Geometry: see drawing. Coordinates: mm, zero at the bounding-box minimum. Round coordinates to 2 decimals unless told otherwise and drop trailing zeros. Loops run counter-clockwise (first coordinate to the right, second up) from the corner with the lowest first, then second, coordinate; pieces in that order, holes last. Notation, with made-up numbers: (89, 82.5) - (139, 82.5) arc R29 ccw to (139, 113.5) - close; hole circle Ø11 at (18, 25). An arc over 180 degrees is marked (long way). Write item = value, one per line. Start each with the question number.
Item 1: Section B-B (x = 14.5). Return loops of the section in (y, z).
Item 2: Section A-A (y = 11). Return loops of the section in (x, z), plus the area to 3 significant figures.
Item 3: Line query: line 1 (Z direction, x = 19, y = 38); line 2 (Z direction, x = 9, y = 12) (1 decimal); line 3 (X direction, y = 4, z = 353). Output: solid intervals per line, ascending. Write a range as from..to.
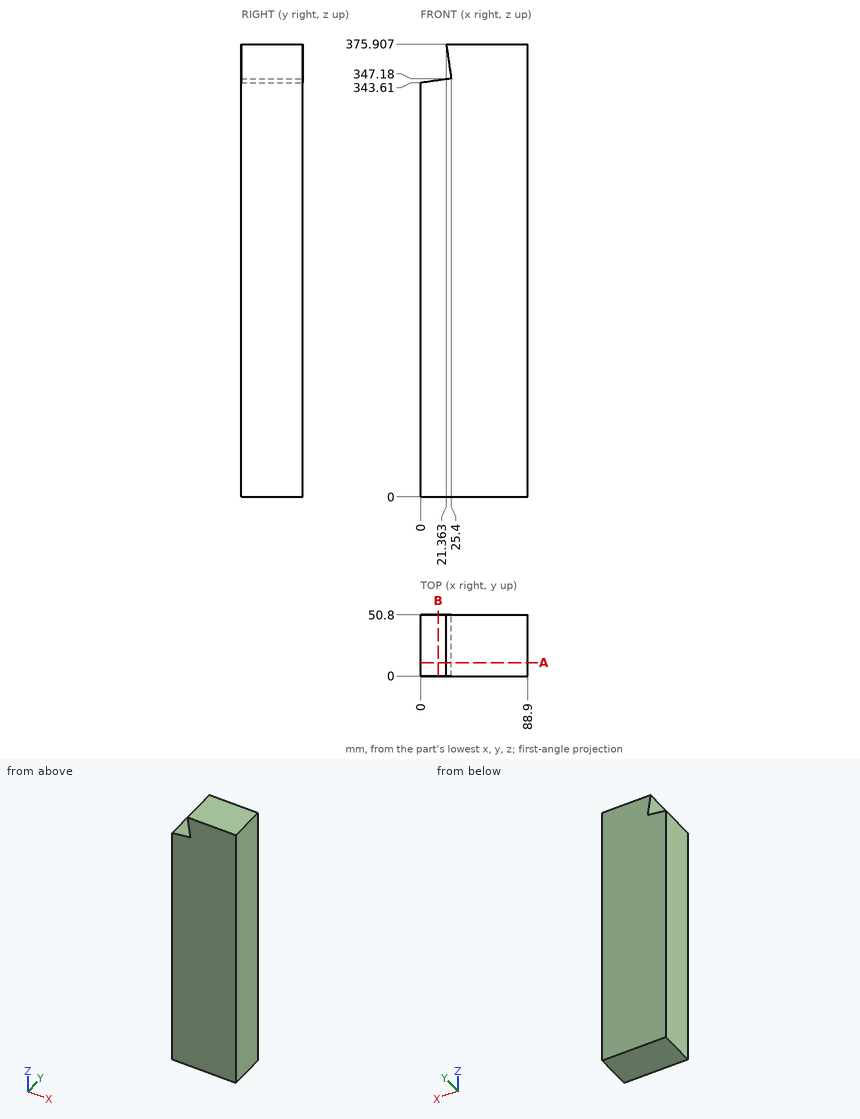
Taken from the geometry:
q1.outline = (0, 0) - (50.8, 0) - (50.8, 345.65) - (0, 345.65) - close
q2.outline = (0, 0) - (88.9, 0) - (88.9, 375.91) - (21.36, 375.91) - (25.4, 347.18) - (0, 343.61) - close
q2.area = 32,700 mm^2
q3.line_1 = 0..346.28
q3.line_2 = 0..344.9
q3.line_3 = 24.58..88.9
